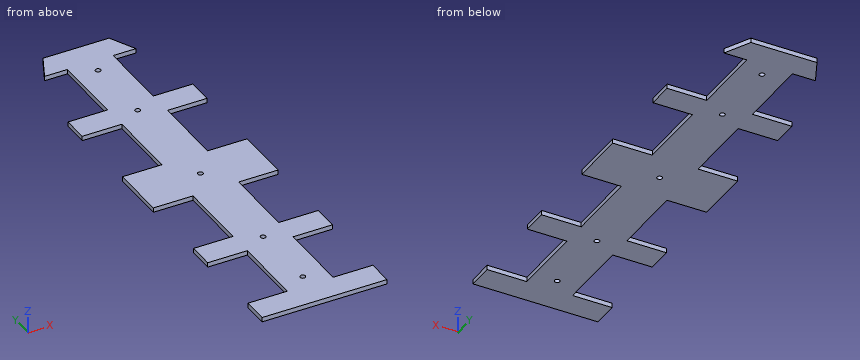
```python
from build123d import *

# Parameters (mm, degrees)
PAD_DEPTH         = 3
SKETCH001_R       = 1.7
POCKET_DEPTH      = 0.001
POCKET_DEPTH_BACK = 3.001


with BuildPart() as part:
    # Sketch → Pad (new body)
    with BuildSketch(Plane.XY):
        Polygon((0, 33), (41, 33), (41, 50), (15, 50), (15, 98), (41, 98), (41, 115), (15, 115), (15, 163), (41, 163), (41, 200), (15, 200), (15, 248), (41, 248), (41, 265), (15, 265), (15, 313), (30, 313), (21.708546, 330), (0, 330), align=None)
    pad = extrude(amount=PAD_DEPTH)

    # Mirrored: Pad across Sketch V_Axis
    add(pad.mirror(Plane(origin=(0, 0, 0), x_dir=(0, 0, 1), z_dir=(1, 0, 0))))

    # Sketch001 → Pocket (cut, two sides)
    with BuildSketch(Plane.XY) as pocket_sk:
        with Locations((0, 59)):
            Circle(SKETCH001_R)
        with Locations((0, 106.3905)):
            Circle(SKETCH001_R)
        with Locations((0, 181.3905)):
            Circle(SKETCH001_R)
        with Locations((0, 256.3905)):
            Circle(SKETCH001_R)
        with Locations((0, 303.7447)):
            Circle(SKETCH001_R)
    extrude(amount=-POCKET_DEPTH, mode=Mode.SUBTRACT)
    extrude(pocket_sk.sketch, amount=POCKET_DEPTH_BACK, mode=Mode.SUBTRACT)


with BuildPart() as part_1:
    # Clone063 placement: moved
    add(part.part.moved(Location((41, -330, 0))))


solid = part_1.part
```
For this review, take the finished solid that the model builds, in its own axes (mm). Round coordinates to 2 decimals unless told otherwise and drop trailing zeros. Write each loop counter-clockwise with the first axis right and the second up, starting at its lowest first coordinate (ties: lowest second). Pieces come first, ordered by that corner, then holes. Notation, with made-up numbers: (51.25, 16.5) -> (105.25, 16.5) arc R6 cw to (105.25, 26.5) -> close; hole circle Ø6 at (45, 77.25). An arc over 180 degrees is marked (long way). Use one line per item in the form item = value.
Q1. Consider section A-A (y = -48). State the section outline as (x, z) points.
Resolved:
outline = (26, 0) -> (56, 0) -> (56, 3) -> (26, 3) -> close
Q2. Clearance check with flat-ended pins moving along their axes: pin 1 Ø1.5 at (y, z) = (-252, 1.5) entering from -X; pin 2 Ø1.5 at (x, z) = (73, 1.5) entering from +Y; pin 3 Ø1.5 at (x, z) = (16, 2) entering from +Y; pin 4 Ø4.5 at (x, y) = (41, -73.61) entering from -Z. State where each tip first meets the part, or that it passes through.
Resolved:
pin_1 = 26
pin_2 = -65
pin_3 = -5.21
pin_4 = 0
Q3. To check wall thickness, follow probe 1 along Y at (x, z) = (41, 2.1); probe 2 along Y at (x, z) = (9, 0.7); probe 3 along Y at (x, z) = (60, 2.6). State the ranges of each line that lie inside material, in increasing order. Write a range as from..to.
Resolved:
probe_1 = -297..-272.7, -269.3..-225.31, -221.91..-150.31, -146.91..-75.31, -71.91..-27.96, -24.56..0
probe_2 = -297..-280, -232..-215, -167..-130, -82..-65
probe_3 = -297..-280, -232..-215, -167..-130, -82..-65, -17..0
Q4. Consider section B-B (z = 2.2). State how many separate pieces and enclosed holes the cut face has, then the cut area to 3 significant figures.
Resolved:
separate_pieces = 1
enclosed_holes = 5
area = 13,800 mm²
